from build123d import *


with BuildPart() as f1:
    # F0 (on Front) → F1 (revolve)
    with BuildSketch(Plane.XZ):
        Polygon((3, 27), (1.5, 27), (1.5, 0), (4.916227, 0), (3, 2.928835), (3, 5.083773), (3, 8.916227), align=None)
        Polygon((4.916227, 7), (3, 8.916227), (3, 5.083773), align=None)
    revolve(axis=Axis((0, 0, 11), (0, 0, 1)))


solid = f1.part
Geometry check sheet. Reference: the model listing, model coordinates, mm. A direction names the side the tool comes from. Round coordinates to 2 decimals unless told otherwise and drop trailing zeros. Order: outer loops, then holes, each group sorted by start corner. A loop starts at its lowest first (then second) coordinate and runs counter-clockwise, first axis right, second up. Notation, with made-up numbers: M 76,47.5 L 100,47.5 A22 cw 100,61.5 Z; hole C -11,-31 d8. An arc over 180 degrees is marked long. Answer in a Markdown table with one row per item. Add a question column.
Item 1: Set-up check for faces 4 (the face through (-0.671, -3.019, 2.787)), 5 (the face through (1.2, 1.2, 0)): record each of +Z, -Z, +X, -X, +Y, -Y from which the full face is reachable in a straight line by a thin tool's end or side.
Item 2: Material ranges on L1, parallel to Y at x = 0, z = 15.5; L2, parallel to Z at x = -3.5, y = 2.75; L3, parallel to X at y = -0.75, z = 23.5, recorded low to high. Write a range as [from, to].
Item 3: Depth check by flat-ended pin: pin 1 Ø5 at (y, z) = (-2, 19) entering from +X; pin 2 Ø3 at (x, z) = (-2, 21) entering from -Y; pin 3 Ø5 at (y, z) = (4, 15) entering from +X. Enter the tip coordinate at first touch or a pass-through.
Item 4: Sectioned sample at A-A, the plane y = 0. Enter the section's corners in (x, z), plus the area to 3 significant figures.
Item 5: Sectioned sample at C-C, the plane z = 24.5. Enter the section's corners in (x, y), plus the area to 3 significant figures.
Item 6: Draft check along Y on faces 1 (the face through (1.3, -1.3, 27)), 2 (the face through (-1.5, 0.07, 13.31)), 3 (the face through (-3, 0, 18)). Enter one of: released by +Y, released by -Y, zero draft, split by the parting line, or undercut.
Filled in:
| question | item | result |
|---|---|---|
| 1 | face 4 | none |
| 1 | face 5 | -Z, +X, -X, +Y, -Y |
| 2 | L1 | y = [-3, -1.5], [1.5, 3] |
| 2 | L2 | z = [0, 0.71], [6.53, 7.47] |
| 2 | L3 | x = [-2.9, -1.3], [1.3, 2.9] |
| 3 | pin 1 | stops at x = 3 |
| 3 | pin 2 | stops at y = -2.96 |
| 3 | pin 3 | stops at x = 2.6 |
| 4 | outline | M -4.92,0 L -1.5,0 L -1.5,27 L -3,27 L -3,8.92 L -4.92,7 L -3,5.08 L -3,2.93 Z; M 1.5,0 L 4.92,0 L 3,2.93 L 3,5.08 L 4.92,7 L 3,8.92 L 3,27 L 1.5,27 Z |
| 4 | area | 94.0 mm² |
| 5 | outline | C 0,0 d6; hole C 0,0 d3 |
| 5 | area | 21.2 mm² |
| 6 | face 1 | zero draft |
| 6 | face 2 | undercut |
| 6 | face 3 | split by the parting line |
